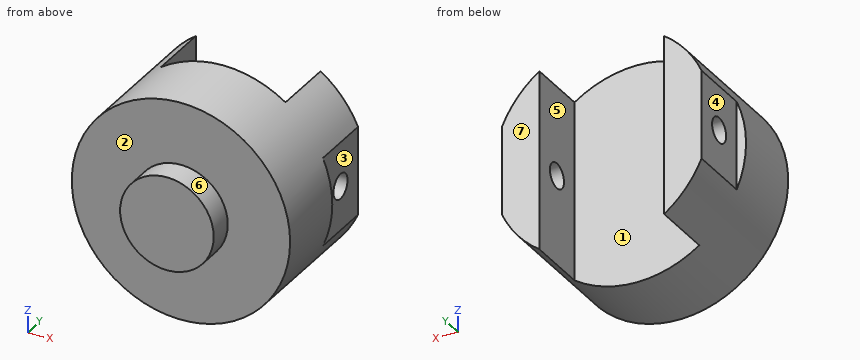
from build123d import *

# Parameters (mm, degrees)
ESBO_O2_W                  = 200
ESBO_O2_H                  = 100
ESBO_O2_W_2                = 15
CORTE_EXTRUS_O1_DEPTH      = 176
CORTE_EXTRUS_O1_DEPTH_BACK = 176
ESBO_O3_R                  = 20
CORTE_EXTRUS_O2_DEPTH      = 16
CORTE_EXTRUS_O2_DEPTH_BACK = 336


with BuildPart() as part:
    # Esboço1 → Revolução1 (revolve)
    with BuildSketch(Plane.XY):
        Polygon((0, 260), (175, 260), (175, 40), (75, 40), (75, 0), (0, 0), align=None)
    revolve(axis=Axis((0, 0, 0), (0, 1, 0)))

    # Esboço2 → Corte-extrusão1 (cut, two sides)
    with BuildSketch(Plane.XY) as corte_extrus_o1_sk:
        with Locations((0, 210)):
            Rectangle(ESBO_O2_W, ESBO_O2_H)
        with Locations((167.5, 210)):
            Rectangle(ESBO_O2_W_2, ESBO_O2_H)
        with Locations((-167.5, 210)):
            Rectangle(ESBO_O2_W_2, ESBO_O2_H)
    extrude(amount=CORTE_EXTRUS_O1_DEPTH, mode=Mode.SUBTRACT)
    extrude(corte_extrus_o1_sk.sketch, amount=-CORTE_EXTRUS_O1_DEPTH_BACK, mode=Mode.SUBTRACT)

    # Esboço3 → Corte-extrusão2 (cut, two sides)
    with BuildSketch(Plane(origin=(160, 0, 0), x_dir=(0, 0, -1), z_dir=(1, 0, 0))) as corte_extrus_o2_sk:
        with Locations((0, 210)):
            Circle(ESBO_O3_R)
    extrude(amount=CORTE_EXTRUS_O2_DEPTH, mode=Mode.SUBTRACT)
    extrude(corte_extrus_o2_sk.sketch, amount=-CORTE_EXTRUS_O2_DEPTH_BACK, mode=Mode.SUBTRACT)


solid = part.part
Read the model definition and answer for the solid it produces. Units are mm, in the model's axes. Face numbers are marked on the shaded views. A direction names the side the tool comes from. Round coordinates to 2 decimals unless told otherwise and drop trailing zeros. Write each loop counter-clockwise with the first axis right and the second up, starting at its lowest first coordinate (ties: lowest second). Pieces come first, ordered by that corner, then holes. Notation, with made-up numbers: (-18.5, 51) - (-10.5, 51) arc R13 ccw to (-10.5, 64) - close; hole circle Ø6 at (53, -6). An arc over 180 degrees is marked (long way). Use a Markdown table: item, result.
(1) The mould has two halves that part along X. Classify the marked faces 5, 6 and 7: released by +X, released by -X, zero draft, split by the parting line, or undercut.
Reported:
| item | result |
|---|---|
| face 5 | undercut |
| face 6 | split by the parting line |
| face 7 | zero draft |
(2) The part is cut by section C-C (x = 0). Write down the section's boundary in (y, z), then the cut area to 3 significant figures.
Reported:
| item | result |
|---|---|
| outline | (0, -75) - (40, -75) - (40, -175) - (160, -175) - (160, 175) - (40, 175) - (40, 75) - (0, 75) - close |
| area | 48,000 mm2 |
(3) Which of the six approach directions +Z, -Z, +X, -X, +Y, -Y give full straight-line access (tool end or side, diameter ignored) to the marked faces 1, 2, 3 and 4?
Reported:
| item | result |
|---|---|
| face 1 | +Z, -Z, +Y |
| face 2 | -Y |
| face 3 | +Z, -Z, +X, +Y |
| face 4 | +Z, -Z, -X, +Y |
(4) The part is cut by section B-B (y = 210). Write down the section's boundary in (x, z), then the cut area to 3 significant figures.
Reported:
| item | result |
|---|---|
| outline | (-160, -70.89) arc R175 ccw to (-100, -143.61) - (-100, -20) - (-160, -20) - close; (-160, 20) - (-100, 20) - (-100, 143.61) arc R175 ccw to (-160, 70.89) - close; (100, -143.61) arc R175 ccw to (160, -70.89) - (160, -20) - (100, -20) - close; (100, 20) - (160, 20) - (160, 70.89) arc R175 ccw to (100, 143.61) - close |
| area | 22,600 mm2 |
(5) The part is cut by section D-D (z = -128.5). Write down the section's boundary in (x, y).
Reported:
| item | result |
|---|---|
| outline | (-118.8, 40) - (118.8, 40) - (118.8, 260) - (100, 260) - (100, 160) - (-100, 160) - (-100, 260) - (-118.8, 260) - close |
(6) The part is cut by section A-A (z = 0). Write down the section's boundary in (x, y).
Reported:
| item | result |
|---|---|
| outline | (-175, 40) - (-75, 40) - (-75, 0) - (75, 0) - (75, 40) - (175, 40) - (175, 160) - (160, 160) - (160, 190) - (100, 190) - (100, 160) - (-100, 160) - (-100, 190) - (-160, 190) - (-160, 160) - (-175, 160) - close; (-160, 230) - (-100, 230) - (-100, 260) - (-160, 260) - close; (100, 230) - (160, 230) - (160, 260) - (100, 260) - close |
(7) Straight lines are drawn through the part: line 1 along X through (y, z) = (209.5, 41); line 2 along Y through (x, z) = (-142, 0); line 3 along X through (y, z) = (30, 24.5). For each, find the intervals that lie inside material, in ascending order. Write a range as [from, to].
Reported:
| item | result |
|---|---|
| line 1 | [-160, -100], [100, 160] |
| line 2 | [40, 190], [230, 260] |
| line 3 | [-70.89, 70.89] |
(8) Each of these flat-tipped pins is pushed along its axis until it touches: pin 1 Ø7.5 at (x, z) = (-170, 6.5) entering from +Y; pin 2 Ø3 at (y, z) = (73.5, -111.5) entering from +X; pin 3 Ø3 at (x, y) = (121, 124.5) entering from -Z. Where does it stop, or does it pass through?
Reported:
| item | result |
|---|---|
| pin 1 | y = 160 |
| pin 2 | x = 136.11 |
| pin 3 | z = -127.85 |
